```python
from build123d import *

# Parameters (mm, degrees)
BOSS_EXTRUDE1_DEPTH = 40
CUT_EXTRUDE1_DEPTH  = 35
FILLET1_R           = 10
BOSS_EXTRUDE2_DEPTH = 3.5
CUT_EXTRUDE5_DEPTH  = 41.96687114982433
BOSS_EXTRUDE3_START = 13.5
BOSS_EXTRUDE3_DEPTH = 13.5
SKETCH10_R          = 2.4999999999999996
CUT_EXTRUDE6_DEPTH  = 13.5
SKETCH11_R          = 4.500000000000001
CUT_EXTRUDE7_DEPTH  = 3
SKETCH12_R          = 1.6339869281045687
CUT_EXTRUDE8_DEPTH  = 44.87521560524114
SHELL3_START        = -0.5
SHELL3_DEPTH        = 1
CUT_EXTRUDE9_DEPTH  = 45.47791075024091


# Read off the part's stored shape, not the designer's step: Shell3
with BuildPart() as part:
    # Sketch1 → Boss-Extrude1 (new body)
    with BuildSketch(Plane.XY):
        Polygon((6.0000000000003, 1.5000000000000038), (6.000000000000302, -1.5), (-6.0000000000000036, -1.5000000000000016), (-6.000000000000004, 1.4999999999999993), align=None)
    extrude(amount=BOSS_EXTRUDE1_DEPTH)

    # Sketch3 → Cut-Extrude1 (cut)
    with BuildSketch(Plane(origin=(6.000000000000301, 3.47e-15, 0), x_dir=(0, 0, -1), z_dir=(1, 5.8e-16, 0))):
        Polygon((-40, 1.5000000000000002), (-36.99999999999992, -1.5000000000000036), (-40, -1.5000000000000036), align=None)
    extrude(amount=-CUT_EXTRUDE1_DEPTH, mode=Mode.SUBTRACT)

    # Fillet1
    fillet1_edges = [part.edges().sort_by_distance(p)[0] for p in [
        (1.4921e-13, -1.5000000000000036, 36.99999999999992),
    ]]
    fillet(fillet1_edges, radius=FILLET1_R)

    # Sketch5 → Boss-Extrude2 (add)
    with BuildSketch(Plane(origin=(-5.4e-16, 1.5000000000000016, 0), x_dir=(1, 3.6e-16, 0), z_dir=(-3.6e-16, 1, 0))):
        with BuildLine():
            Line((6.000000000000301, -17.495666027521235), (6.000000000000301, -34.00043164524958))
            ThreePointArc((6.000000000000301, -34.00043164524958), (3.235e-14, -40.00043164524985), (-6.000000000000234, -34.00043164524958))
            Line((-6.000000000000234, -34.00043164524958), (-6.000000000000234, -17.495666027521235))
            ThreePointArc((-6.000000000000234, -17.495666027521235), (3.382e-14, -11.495666027520969), (6.000000000000301, -17.495666027521235))
        make_face()
    extrude(amount=BOSS_EXTRUDE2_DEPTH)

    # Sketch8 → Cut-Extrude5 (cut, through all)
    with BuildSketch(Plane(origin=(-1.81e-15, 5.000000000000002, 0), x_dir=(1, 3.6e-16, 0), z_dir=(-3.6e-16, 1, 0))):
        with BuildLine():
            Line((-6.000000000000004, -40), (-0.07196913699948215, -40))
            ThreePointArc((-0.07196913699948213, -40.00000000000001), (-4.268009771661707, -38.217550636812796), (-6.000000000000242, -34.00043164524961))
            Line((-6.0000000000002425, -34.00043164524961), (-6.000000000000004, -40))
        make_face()
        with BuildLine():
            ThreePointArc((6.000000000000299, -34.00043164524958), (4.268009771661984, -38.217550636812554), (0.07196913700016037, -40))
            Line((0.07196913700015983, -40), (6.000000000000301, -40))
            Line((6.000000000000301, -40), (6.000000000000301, -34.00043164524958))
        make_face()
    extrude(amount=-CUT_EXTRUDE5_DEPTH, mode=Mode.SUBTRACT)

    # Sketch9 → Boss-Extrude3 (add)
    with BuildSketch(Plane(origin=(-1.81e-15, 5.000000000000002, 0), x_dir=(1, 3.6e-16, 0), z_dir=(-3.6e-16, 1, 0)).offset(BOSS_EXTRUDE3_START)):
        with BuildLine():
            Line((-6.000000000000234, -29.081568785258), (6.000000000000301, -29.081568785258))
            Line((6.000000000000301, -29.081568785258), (6.000000000000301, -34.00043164524958))
            ThreePointArc((6.000000000000301, -34.00043164524958), (3.272e-14, -40.00043164524985), (-6.000000000000234, -34.00043164524958))
            Line((-6.000000000000234, -34.00043164524958), (-6.000000000000234, -29.081568785258))
        make_face()
    extrude(amount=-BOSS_EXTRUDE3_DEPTH)

    # Sketch10 → Cut-Extrude6 (cut)
    with BuildSketch(Plane(origin=(-1.81e-15, 5.000000000000002, 0), x_dir=(1, 3.6e-16, 0), z_dir=(-3.6e-16, 1, 0))):
        with Locations(Location((1e-17, -17.403956104439153, 0), (0, 0, 180))):
            Circle(SKETCH10_R)
    extrude(amount=-CUT_EXTRUDE6_DEPTH, mode=Mode.SUBTRACT)

    # Sketch11 → Cut-Extrude7 (cut)
    with BuildSketch(Plane(origin=(-1.81e-15, 5.000000000000002, 0), x_dir=(1, 3.6e-16, 0), z_dir=(-3.6e-16, 1, 0))):
        with Locations(Location((1e-17, -17.403956104439153, 0), (0, 0, 180))):
            Circle(SKETCH11_R)
    extrude(amount=-CUT_EXTRUDE7_DEPTH, mode=Mode.SUBTRACT)

    # Sketch12 → Cut-Extrude8 (cut, through all)
    with BuildSketch(Plane(origin=(-5.4e-16, 1.5000000000000016, 0), x_dir=(1, 3.6e-16, 0), z_dir=(-3.6e-16, 1, 0))):
        with Locations((1e-17, -17.403956104439153)):
            Circle(SKETCH12_R)
        with BuildLine():
            Line((1.6350000000000315, -8.142419448359679), (1.6350000000000313, -6.270656428732565))
            ThreePointArc((1.6350000000000313, -6.270656428732565), (0.00101307189543799, -4.636669500627991), (-1.6329738562091354, -6.270656428732585))
            Line((-1.6329738562091354, -6.270656428732585), (-1.6329738562091352, -8.110833214748085))
            ThreePointArc((-1.6329738562091352, -8.110833214748085), (-0.01582557591703412, -9.86878595405819), (1.6350000000000315, -8.142419448359679))
        make_face()
    extrude(amount=-CUT_EXTRUDE8_DEPTH, mode=Mode.SUBTRACT)

    # Shell3 outline → Shell3 (cut)
    with BuildSketch(Plane.YZ.offset(SHELL3_START)):
        with BuildLine():
            Line((4, 29.081568785), (13, 29.081568785))
            Line((13, 29.081568785), (13, 32.857864376))
            ThreePointArc((13, 32.857864376), (8.5, 37.357864376), (4, 32.857864376))
            Line((4, 32.857864376), (4, 29.081568785))
        make_face()
    extrude(amount=SHELL3_DEPTH, mode=Mode.SUBTRACT)

    # Sketch18 → Cut-Extrude9 (cut, through all)
    with BuildSketch(Plane(origin=(0, 0, 0), x_dir=(-1, 0, 0), z_dir=(0, 0, -1))):
        Polygon((6.000000000000441, 1.5), (6.000000000000442, -1.499999999999904), (-5.999999999999879, -1.4999999999999782), (-5.999999999999879, 1.5000000000000229), (-4.000000000000168, 1.5000000000001654), (-4.000000000000022, 2.5000000000001656), (-7.000000000000024, 2.500000000000053), (-7.000000000000022, -2.499999999999947), (7, -2.4999999999998628), (6.999999999999999, 2.500000000000055), (4.000000000000475, 2.5000000000000546), (4.000000000000459, 1.5), align=None)
    extrude(amount=-CUT_EXTRUDE9_DEPTH, mode=Mode.SUBTRACT)


solid = part.part
```
Geometry: final body of the model. Coordinates: model frame, mm. A direction names the side the tool comes from. Coordinates: 2 decimals unless noted, no trailing zeros. Order: outer loops, then holes, each group sorted by start corner. A loop starts at its lowest first (then second) coordinate and runs counter-clockwise, first axis right, second up. Notation, with made-up numbers: (15.5, -13.75) - (33.5, -13.75) arc R24 cw to (33.5, -3.75) - close; hole circle Ø2 at (9.25, -22). An arc over 180 degrees is marked (long way). Write each question's results on one line, items separated by ' | '.
1) Section C-C, the plane z = 35.5. Return loops of the section in (x, y), plus the area to 3 significant figures.
Results list:
outline: (-5.81, -1.14) - (5.81, -1.14) - (5.81, 1.5) - (4, 1.5) - (4, 2.5) - (5.81, 2.5) - (5.81, 18.5) - (-5.81, 18.5) - (-5.81, 2.5) - (-4, 2.5) - (-4, 1.5) - (-5.81, 1.5) - close; hole (-0.5, 4.86) - (0.5, 4.86) - (0.5, 12.14) - (-0.5, 12.14) - close | area: 217 mm^2
2) Pin query (flat end, axial travel): pin 1 (3 mm diameter, centred on x = -3.5, z = 22, fed in from +Y); pin 2 (0.8 mm diameter, centred on y = 2, z = 21, fed in from +X); pin 3 (4 mm diameter, centred on x = 1.5, y = 6, fed in from -Z); pin 4 (4.5 mm diameter, centred on x = 0, z = 17.4, fed in from -Y). Return the tip coordinate at first contact, or that it passes through.
Results list:
pin 1: y = 5 | pin 2: x = 4 | pin 3: z = 11.5 | pin 4: through
3) Section A-A, the plane y = 8.5. Return loops of the section in (x, z), plus the area to 3 significant figures.
Results list:
outline: (-6, 29.08) - (-0.5, 29.08) - (-0.5, 37.36) - (0.5, 37.36) - (0.5, 29.08) - (6, 29.08) - (6, 34) arc R6 ccw to (-6, 34) - close | area: 107 mm^2
4) Pull-direction query (Y, two-part tool) for faces 1 (the flat face through (-5, 2.5, 26)), 2 (the flat face through (0, 4.5, 29.082)), 3 (the flat face through (0, 18.5, 34)), 4 (the flat face through (6, 0, 17)); classes: pulls with the +Y half, pulls with the -Y half, needs draft (parallel to the pull), parting line crosses it, or undercut.
Results list:
face 1: undercut | face 2: undercut | face 3: pulls with the +Y half | face 4: needs draft
5) Set-up query: faces 5 (the flat face through (3, 2, 17)), 6 (the cylindrical face through (-0.132, 3.614, 11.497)), 7 (the flat face through (0, 13, 31)). Return all of +Z, -Z, +X, -X, +Y, -Y with unobstructed straight access to the full face (end or side cutting, diameter ignored); none if empty.
Results list:
face 5: +Y | face 6: -Z, +Y | face 7: -Z
6) Section D-D, the plane z = 11. Return loops of the section in (x, y), plus the area to 3 significant figures.
Results list:
outline: (-6, -1.5) - (6, -1.5) - (6, 1.5) - (-6, 1.5) - close | area: 36.0 mm^2
7) Section B-B, the plane x = 5.25. Return loops of the section in (y, z).
Results list:
outline: (-1.5, 0) - (1.5, 0) - (1.5, 36.91) - (-0.64, 36.91) arc R10 ccw to (-1.5, 32.86) - close; (2.5, 14.59) - (5, 14.59) - (5, 29.08) - (18.5, 29.08) - (18.5, 36.91) - (2.5, 36.91) - close
8) Line query: line 1 (Y direction, x = 4.25, z = 13.5); line 2 (Z direction, x = 0, y = 3.9); line 3 (Z direction, x = 0, y = -0.65). Output: solid intervals per line, ascending. Write a range as from..to.
Results list:
line 1: -1.5..1.5, 2.5..5 | line 2: 11.5..12.9, 21.9..40 | line 3: 0..4.64, 9.87..14.9, 19.9..36.89
